from build123d import *

# Parameters (mm, degrees)
SKETCH_1_W          = 55.4
SKETCH_1_H          = 13
SKETCH_1_R          = 1.5
SKETCH_1_W_2        = 44
SKETCH_1_H_2        = 4.8
EXTRUDE_1_DEPTH     = 1
SKETCH_2_W          = 55.4
SKETCH_2_H          = 1
EXTRUDE_2_DEPTH     = 10.75
CUT_EXTRUDE_1_DEPTH = 2
SKETCH_4_R          = 1.5
CUT_EXTRUDE_2_DEPTH = 2
FILLET_1_R          = 0.5
FILLET_2_R          = 1
FILLET_3_R          = 1.5
FILLET_4_R          = 1


with BuildPart() as part:
    # 草图1 → 凸台-拉伸1 (new body)
    with BuildSketch(Plane.XY):
        with Locations((0, 6.5)):
            Rectangle(SKETCH_1_W, SKETCH_1_H)
        with Locations((-24.5, 3)):
            Circle(SKETCH_1_R, mode=Mode.SUBTRACT)
        with Locations((24.5, 3)):
            Circle(SKETCH_1_R, mode=Mode.SUBTRACT)
        with Locations((0, 5.9)):
            Rectangle(SKETCH_1_W_2, SKETCH_1_H_2, mode=Mode.SUBTRACT)
    extrude(amount=EXTRUDE_1_DEPTH)

    # 草图2 → 凸台-拉伸2 (add)
    with BuildSketch(Plane.XY.offset(1)):
        with Locations((0, 12.5)):
            Rectangle(SKETCH_2_W, SKETCH_2_H)
    extrude(amount=EXTRUDE_2_DEPTH)

    # 草图3 → 切除-拉伸1 (cut, through all)
    with BuildSketch(Plane.XZ.offset(-12)):
        Polygon((-27.7, 11.75), (-27.7, 7), (-10, 11.75), align=None)
        Polygon((27.7, 11.75), (27.7, 7), (10, 11.75), align=None)
    extrude(amount=-CUT_EXTRUDE_1_DEPTH, mode=Mode.SUBTRACT)

    # 草图4 → 切除-拉伸2 (cut, through all)
    with BuildSketch(Plane.XZ.offset(-12)):
        with Locations((-5, 8.25)):
            Circle(SKETCH_4_R)
        with Locations((5, 8.25)):
            Circle(SKETCH_4_R)
    extrude(amount=-CUT_EXTRUDE_2_DEPTH, mode=Mode.SUBTRACT)

    # 圆角1
    fillet_1_edges = [part.edges().sort_by_distance(p)[0] for p in [
        (0, 13, 0),
        (0, 12, 1),
    ]]
    fillet(fillet_1_edges, radius=FILLET_1_R)

    # 圆角2
    fillet_2_edges = [part.edges().sort_by_distance(p)[0] for p in [
        (22, 3.5, 0.5),
        (22, 8.3, 0.5),
        (-22, 8.3, 0.5),
        (-22, 3.5, 0.5),
    ]]
    fillet(fillet_2_edges, radius=FILLET_2_R)

    # 圆角3
    fillet_3_edges = [part.edges().sort_by_distance(p)[0] for p in [
        (27.7, 0, 0.5),
        (-27.7, 0, 0.5),
    ]]
    fillet(fillet_3_edges, radius=FILLET_3_R)

    # 圆角4
    fillet_4_edges = [part.edges().sort_by_distance(p)[0] for p in [
        (-27.7, 12.5, 7),
        (27.7, 12.5, 7),
    ]]
    fillet(fillet_4_edges, radius=FILLET_4_R)


solid = part.part
Design review of the part built by this model. Coordinates are the model's own, in mm. A direction names the side the tool comes from. Round coordinates to 2 decimals unless told otherwise and drop trailing zeros. Write each loop counter-clockwise with the first axis right and the second up, starting at its lowest first coordinate (ties: lowest second). Pieces come first, ordered by that corner, then holes.
Item 1: Consider section B-B on y = 3. Give the boundary of the cut face in (x, z), and give its area (3 significant figures).
Item 2: For pin 1 Ø3 at (x, y) = (-14.5, 4.5) entering from -Z; pin 2 Ø3.5 at (x, y) = (24.5, 3) entering from +Z; pin 3 Ø1.8 at (x, y) = (-24.5, 3) entering from -Z; pin 4 Ø5 at (x, z) = (-5, 8.25) entering from -Y, all flat-tipped, find the tip position at first contact; note any pin that passes through.
Item 3: Wall thickness on L1, parallel to Z at x = -5, y = 12.3; L2, parallel to Y at x = 24.5, z = 0.65; L3, parallel to Y at x = 16, z = 0.5: over which ranges is each line inside the solid? List them lowest first.
Item 4: Consider section C-C on z = 8.25. Give the boundary of the cut face in (x, y).
Item 5: Consider section A-A on x = 5. Give the boundary of the cut face in (y, z), and give its area (4 significant figures).
Item 6: Draft analysis for pull direction Z (two halves, no side actions). For faces 4 (the cylindrical face through (5.69, 12.49, 6.92)), 5 (the flat face through (0, 12, 5)), 6 (the cylindrical face through (-27.5, 12.51, 6.83)), state which applies: released by +Z, released by -Z, zero draft, split by the parting line, or undercut.
Item 7: For faces 1 (the flat face through (-0.4, 0, 0.5)), 2 (the flat face through (0, 3, 1)), 3 (the flat face through (-22, 5.9, 0.5)), list the 3-axis set-ups (+Z, -Z, +X, -X, +Y, -Y) from which the entire face can be reached by the end or side of a thin tool; tool diameter is ignored.
Item 8: Consider section D-D on x = -11.5. Give the boundary of the cut face in (y, z), and give its area (3 significant figures).
Check values:
1. outline: (-27.7, 0) - (-26, 0) - (-26, 1) - (-27.7, 1) - close; (-23, 0) - (23, 0) - (23, 1) - (-23, 1) - close; (26, 0) - (27.7, 0) - (27.7, 1) - (26, 1) - close
1. area: 49.4 mm2
2. pin 1: stops at z = 0
2. pin 2: stops at z = 1
2. pin 3: passes through
2. pin 4: stops at y = 12
3. L1: z = 0 to 6.75, 9.75 to 11.75
3. L2: y = 0 to 1.5, 4.5 to 13
3. L3: y = 0 to 3.5, 8.3 to 13
4. outline: (-23.04, 12) - (-6.5, 12) - (-6.5, 13) - (-23.04, 13) - close; (-3.5, 12) - (3.5, 12) - (3.5, 13) - (-3.5, 13) - close; (6.5, 12) - (23.04, 12) - (23.04, 13) - (6.5, 13) - close
5. outline: (0, 0) - (3.5, 0) - (3.5, 1) - (0, 1) - close; (8.3, 0) - (12.5, 0) arc R0.5 ccw to (13, 0.5) - (13, 6.75) - (12, 6.75) - (12, 1.5) arc R0.5 cw to (11.5, 1) - (8.3, 1) - close; (12, 9.75) - (13, 9.75) - (13, 11.75) - (12, 11.75) - close
5. area: 15.95 mm2
6. face 4: undercut
6. face 5: zero draft
6. face 6: released by +Z
7. face 1: +Z, -Z, +X, -X, -Y
7. face 2: +Z, +X, -X, -Y
7. face 3: +Z, -Z
8. outline: (0, 0) - (3.5, 0) - (3.5, 1) - (0, 1) - close; (8.3, 0) - (12.5, 0) arc R0.5 ccw to (13, 0.5) - (13, 11.35) - (12, 11.35) - (12, 1.5) arc R0.5 cw to (11.5, 1) - (8.3, 1) - close
8. area: 18.5 mm2
